```python
from build123d import *

# Parameters (mm, degrees)
BOSS_EXTRUDE1_DEPTH     = 1.5875
F_1_4_CLEARANCE_HOLE1_D = 6.5278


with BuildPart() as part:
    # Sketch1 → Boss-Extrude1 (new body)
    with BuildSketch(Plane.XY):
        with BuildLine():
            ThreePointArc((7.267638826, 3.191446717), (0, 7.9375), (-7.267638826, 3.191446717))
            Line((-7.267638826, 3.191446717), (-10.968425472, -5.236073182))
            Line((-10.968425472, -5.236073182), (-9.514897707, -5.874362525))
            Line((-9.514897707, -5.874362525), (-13.344633767, -14.595529116))
            Line((-13.344633767, -14.595529116), (-14.798161533, -13.957239773))
            Line((-14.798161533, -13.957239773), (-25.4, -38.1))
            Line((-25.4, -38.1), (25.4, -38.1))
            Line((25.4, -38.1), (14.798161533, -13.957239773))
            Line((14.798161533, -13.957239773), (13.344633767, -14.595529116))
            Line((13.344633767, -14.595529116), (9.514897707, -5.874362525))
            Line((9.514897707, -5.874362525), (10.968425472, -5.236073182))
            Line((10.968425472, -5.236073182), (7.267638826, 3.191446717))
        make_face()
    extrude(amount=BOSS_EXTRUDE1_DEPTH)

    # 1/4 Clearance Hole1 (through all)
    with Locations(Plane.XY.offset(1.5875)):
        with Locations((0, 0)):
            Hole(F_1_4_CLEARANCE_HOLE1_D / 2)


solid = part.part
```
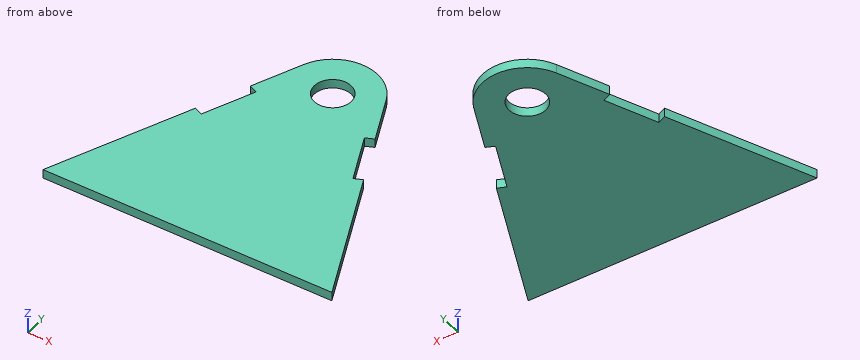
Here's how the part is built. I have some questions about the finished solid (model axes, mm). Round coordinates to 2 decimals unless told otherwise and drop trailing zeros. Write each loop counter-clockwise with the first axis right and the second up, starting at its lowest first coordinate (ties: lowest second). Pieces come first, ordered by that corner, then holes.
Q1. If we section it at C-C on y = 0: Write out the boundary of the cut face in (x, z).
Q2. Please list where these lines run through material, in increasing order: probe 1 along Y at (x, z) = (0, 0.9); probe 2 along Y at (x, z) = (-1, 1.3); probe 3 along X at (y, z) = (-26.5, 1).
Q3. If we section it at D-D on y = -28.5: Write out the boundary of the cut face in (x, z).
Q4. If we section it at B-B on x = 0: Write out the boundary of the cut face in (y, z), plus the area to 3 significant figures.
Q5. If we section it at A-A on z = 1.1: Write out the boundary of the cut face in (x, y) (1 decimal).
Answer below:
1. outline: (-8.67, 0) - (-3.26, 0) - (-3.26, 1.59) - (-8.67, 1.59) - close; (3.26, 0) - (8.67, 0) - (8.67, 1.59) - (3.26, 1.59) - close
2. probe 1: y = -38.1 to -3.26, 3.26 to 7.94
2. probe 2: y = -38.1 to -3.11, 3.11 to 7.87
2. probe 3: x = -20.31 to 20.31
3. outline: (-21.18, 0) - (21.18, 0) - (21.18, 1.59) - (-21.18, 1.59) - close
4. outline: (-38.1, 0) - (-3.26, 0) - (-3.26, 1.59) - (-38.1, 1.59) - close; (3.26, 0) - (7.94, 0) - (7.94, 1.59) - (3.26, 1.59) - close
4. area: 62.7 mm2
5. outline: (-25.4, -38.1) - (25.4, -38.1) - (14.8, -14) - (13.3, -14.6) - (9.5, -5.9) - (11, -5.2) - (7.3, 3.2) arc R7.9 ccw to (-7.3, 3.2) - (-11, -5.2) - (-9.5, -5.9) - (-13.3, -14.6) - (-14.8, -14) - close; hole circle Ø6.5 at (0, 0)
